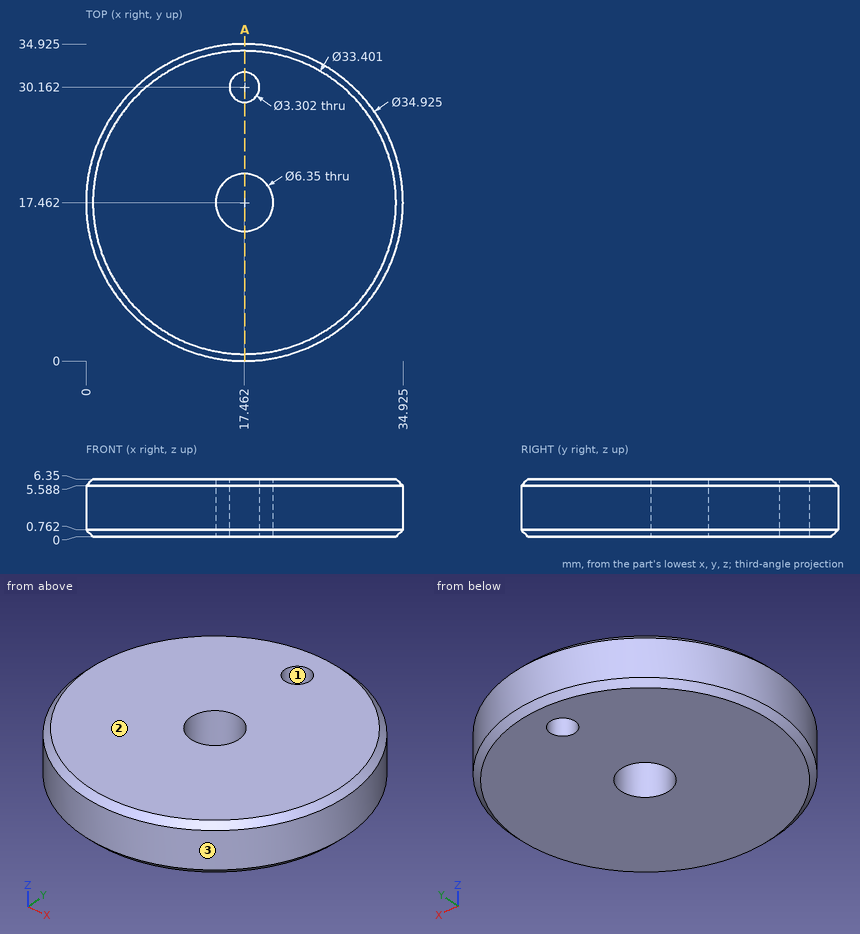
Could you check a few things on this drawing? It's one solid part, dimensions in mm from its lowest x, y, z. Coordinates: 2 decimals unless noted, no trailing zeros.
1) We'd pull the mould along Y, two halves only. Please class the marked faces 1, 2 and 3: +Y half, -Y half, draft (parallel to the pull), parting line (faces both ways), or undercut.
2) Imagine slicing it at A-A on x = 17.5. State how many separate pieces and enclosed holes the cut face has, and give its area (3 significant figures).
3) I need wall thicknesses on line 1 (Y direction, x = 17.5, z = 5) (1 decimal); line 2 (Y direction, x = 16.5, z = 4) (1 decimal); line 3 (X direction, y = 19, z = 6) (1 decimal). Which ranges of each line are inside material? Lowest first, please.
4) Will these pins go through, and if not, where does the flat tip stop? pin 1 (1 mm diameter, centred on y = 26.5, z = 3.5, fed in from -X); pin 2 (3 mm diameter, centred on x = 17.46, y = 30.16, fed in from +Z); pin 3 (1 mm diameter, centred on y = 30.5, z = 4.5, fed in from -X); pin 4 (3 mm diameter, centred on y = 15, z = 2.5, fed in from -X).
Response values:
1. face 1: undercut
1. face 2: draft
1. face 3: parting line
2. separate pieces: 3
2. enclosed holes: 0
2. area: 159 mm2
3. line 1: y = 0 to 14.3, 20.6 to 28.5, 31.8 to 34.9
3. line 2: y = 0 to 14.4, 20.5 to 28.8, 31.5 to 34.9
3. line 3: x = 0.5 to 14.7, 20.2 to 34.4
4. pin 1: stops at x = 2.23
4. pin 2: passes through
4. pin 3: stops at x = 5.31
4. pin 4: stops at x = 0.03
